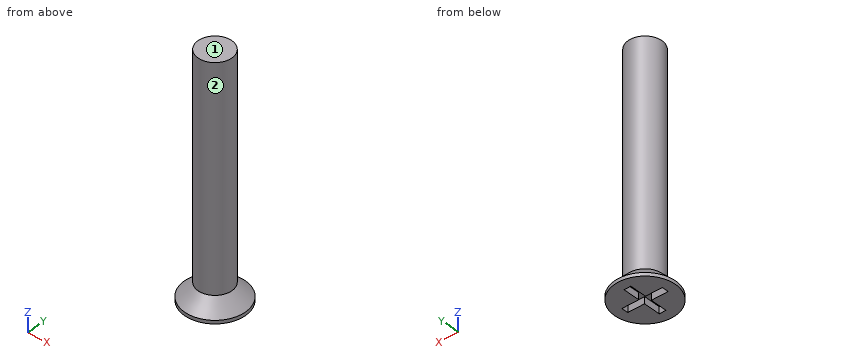
Autodesk Inventor part; units mm, degrees
ref_plane "YZ Plane" through (0, 0, 0) normal (1, 0, 0) x (0, 1, 0)
ref_plane "XZ Plane" through (0, 0, 0) normal (0, 1, 0) x (-1, 0, 0)
ref_plane "XY Plane" through (0, 0, 0) normal (0, 0, 1) x (1, 0, 0)
sketch "Эскиз1" plane through (0, 0, 0) normal (0, 0, 1) x (1, 0, 0)
  circle A0 centre (0, 0) radius 4.5
  dimension "d0" = 9
extrude "Выдавливание1" add sketch "Эскиз1" along normal blind 2.5
sketch "Эскиз2" plane through (0, 0, 2.5) normal (0, 0, 1) x (1, 0, 0)
  circle A0 centre (0, 0) radius 2.5
  dimension "d3" = 5
extrude "Выдавливание2" add sketch "Эскиз2" along normal blind 32.5
chamfer "Фаска1" distance 2 angle 45 1 edges at (-4.5, 0, 2.5)
thread "Резьба1"
sketch "Эскиз3" plane through (0, 0, 0) normal (0, 0, -1) x (-1, 0, 0)
  line L0 (-3, 0.5) -> (3, 0.5)
  line L1 (3, 0.5) -> (3, -0.5)
  line L2 (3, -0.5) -> (-3, -0.5)
  line L3 (-3, -0.5) -> (-3, 0.5)
  line L4 (-0.5, 3) -> (0.5, 3)
  line L5 (0.5, 3) -> (0.5, -3)
  line L6 (0.5, -3) -> (-0.5, -3)
  line L7 (-0.5, -3) -> (-0.5, 3)
  line L8 (0, 3) -> (0, -3) construction
  line L9 (-3, 0) -> (3, 0) construction
  point P0 (0, 0)
  point P1 (0, 0)
  point P2 (-0.5, 0.5)
  point P3 (-0.5, -0.5)
  point P4 (0.5, 0.5)
  point P5 (0.5, -0.5)
  dimension "d12" = 1
  dimension "d13" = 6
extrude "Выдавливание3" cut sketch "Эскиз3" against normal blind 1
properties part number "Болт М5х35"
Geometry: final body of the model. Coordinates: model frame, mm. Face numbers are marked on the shaded views. A direction names the side the tool comes from. Round coordinates to 2 decimals unless told otherwise and drop trailing zeros. Order: outer loops, then holes, each group sorted by start corner. A loop starts at its lowest first (then second) coordinate and runs counter-clockwise, first axis right, second up. Notation, with made-up numbers: M 65.5,-2.5 L 101.5,-2.5 A23 ccw 101.5,13.5 Z; hole C 44,-34.75 d3. An arc over 180 degrees is marked long. Use one line per item in the form item = value. Start each with the question number.
Q1. Pin query (flat end, axial travel): pin 1 Ø0.5 at (y, z) = (1.5, 0.5) entering from +X; pin 2 Ø0.8 at (y, z) = (-2, 0.5) entering from +X; pin 3 Ø3 at (y, z) = (3.5, 30.5) entering from +X. Return the tip coordinate at first contact, or that it passes through.
Q2. Material intervals for line 1 (X direction, y = 2.25, z = 18.5); line 2 (Y direction, x = 0.75, z = 15); line 3 (Y direction, x = -2, z = 17.5), sorted ascending. Write a range as [from, to].
Q3. Cut plane C-C (z = 12). Return loops of the section in (x, y).
Q4. Access query for the marked faces 1 and 2. Directions: +Z, -Z, +X, -X, +Y, -Y. A direction counts if a zero-diameter tool reaches every point of the face in a straight line with its end or side. Return the directions, or none.
Geometry results:
q1.pin_1 = 4.32
q1.pin_2 = 4.21
q1.pin_3 = 1.5
q2.line_1 = [-1.09, 1.09]
q2.line_2 = [-2.38, 2.38]
q2.line_3 = [-1.5, 1.5]
q3.outline = C 0,0 d5
q4.face_1 = +Z, +X, -X, +Y, -Y
q4.face_2 = +Z
